Input: part model. Units: mm. Frame: model coordinates. Face numbers are marked on the shaded views. A direction names the side the tool comes from. Give positions to 0.01 mm unless a question says otherwise; leave off trailing zeros. Order: outer loops, then holes, each group sorted by start corner. A loop starts at its lowest first (then second) coordinate and runs counter-clockwise, first axis right, second up.
```python
from build123d import *

# Parameters (mm, degrees)
BOSS_EXTRUDE1_DEPTH = 56.45658
BOSS_EXTRUDE2_DEPTH = 6.2738
BOSS_EXTRUDE3_DEPTH = 6.2738
SKETCH5_R           = 3.1369
CUT_EXTRUDE1_DEPTH  = 22.95576
SKETCH6_R           = 7.05612
CUT_EXTRUDE2_DEPTH  = 53.31968


with BuildPart() as part:
    # Sketch1 → Boss-Extrude1 (new body)
    with BuildSketch(Plane(origin=(0, 0, 0), x_dir=(0, 0, -1), z_dir=(1, 0, 0))):
        with BuildLine():
            Line((10.97788, 10.97788), (10.97788, -10.97788))
            Line((10.97788, -10.97788), (9.4107, -10.97788))
            Line((9.4107, -10.97788), (9.4107, -9.4107))
            Line((9.4107, -9.4107), (0, -9.4107))
            ThreePointArc((0, -9.4107), (-9.4107, 0), (0, 9.4107))
            Line((0, 9.4107), (9.4107, 9.4107))
            Line((9.4107, 9.4107), (9.4107, 10.97788))
            Line((9.4107, 10.97788), (10.97788, 10.97788))
        make_face()
    extrude(amount=-BOSS_EXTRUDE1_DEPTH)

    # Sketch3 → Boss-Extrude2 (add)
    with BuildSketch(Plane(origin=(-1.56718, 0, 0), x_dir=(0, 0, -1), z_dir=(1, 0, 0))):
        with BuildLine():
            Line((9.4107, 10.97788), (0, 10.97788))
            ThreePointArc((0, 10.97788), (-10.97788, 0), (0, -10.97788))
            Line((0, -10.97788), (9.4107, -10.97788))
            Line((9.4107, -10.97788), (9.4107, 10.97788))
        make_face()
    extrude(amount=-BOSS_EXTRUDE2_DEPTH)

    # Sketch4 → Boss-Extrude3 (add)
    with BuildSketch(Plane(origin=(0, 10.97788, 0), x_dir=(1, 0, 0), z_dir=(0, 1, 0))):
        with BuildLine():
            Line((-56.45658, 10.97788), (-65.86728, 10.97788))
            ThreePointArc((-65.86728, 10.97788), (-72.521649786, -5.087189786), (-56.45658, 1.56718))
            Line((-56.45658, 1.56718), (-56.45658, 10.97788))
        make_face()
    boss_extrude3 = extrude(amount=-BOSS_EXTRUDE3_DEPTH)

    # Mirror1: Boss-Extrude3 across plane
    add(boss_extrude3.mirror(Plane.ZX))

    # Sketch5 → Cut-Extrude1 (cut, through all)
    with BuildSketch(Plane(origin=(0, 10.97788, 0), x_dir=(1, 0, 0), z_dir=(0, 1, 0))):
        with Locations((-65.86728, 1.56718)):
            Circle(SKETCH5_R)
    extrude(amount=-CUT_EXTRUDE1_DEPTH, mode=Mode.SUBTRACT)

    # Sketch6 → Cut-Extrude2 (cut)
    with BuildSketch(Plane(origin=(0, 0, 0), x_dir=(0, 0, -1), z_dir=(1, 0, 0))):
        Circle(SKETCH6_R)
    extrude(amount=-CUT_EXTRUDE2_DEPTH, mode=Mode.SUBTRACT)


solid = part.part
```
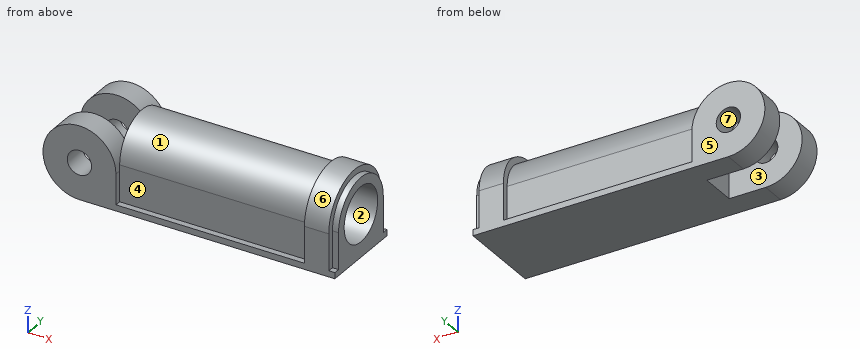
1) Cut plane B-B (y = -1). Return the cut outline in (x, z), then the cut area to 3 significant figures.
2) Reachability of the marked faces 1, 2, 3 and 4 from +Z, -Z, +X, -X, +Y, -Y: full face, straight path, thin tool, end or side. Return the list, or none.
3) Cut plane A-A (x = -15.5). Return the cut outline in (y, z), then the cut area to 3 significant figures.
4) Cut plane D-D (x = -68). Return the cut outline in (y, z), then the cut area to 3 significant figures.
5) Pull-direction query (Z, two-part tool) for the marked faces 5, 6 and 7; classes: pulls with the +Z half, pulls with the -Z half, needs draft (parallel to the pull), parting line crosses it, or undercut.
6) First-contact query: P1, Ø12, axis at x = -52, y = 4.5, coming from the +Z side; P2, Ø4, axis at x = -39.5, y = -7.5, coming from the +Z side; P3, Ø0.8, axis at y = 10, z = -7, coming from the +X side. Flat tips, straight axial feed; report the tip coordinate or a pass-through.
7) Cut plane C-C (z = -5.75). Return the cut outline in (x, y), then the cut area to 3 significant figures.
8) Line query: probe 1 along Y at (x, z) = (-36, 0); probe 2 along Y at (x, z) = (-65, -5); probe 3 along X at (y, z) = (9.5, 1.25). Output: solid intervals per line, ascending.
Geometry says:
1. outline: (-56.46, -10.98) - (0, -10.98) - (0, -6.98) - (-53.32, -6.98) - (-53.32, 6.98) - (0, 6.98) - (0, 9.36) - (-1.57, 9.36) - (-1.57, 10.93) - (-7.84, 10.93) - (-7.84, 9.36) - (-56.46, 9.36) - close
1. area: 413 mm2
2. face 1: +Z
2. face 2: +X
2. face 3: +Z, -Z, -X
2. face 4: +Z, -Y
3. outline: (-10.98, -10.98) - (10.98, -10.98) - (10.98, -9.41) - (9.41, -9.41) - (9.41, 0) arc R9.41 ccw to (-9.41, 0) - (-9.41, -9.41) - (-10.98, -9.41) - close; hole circle Ø14.11 at (0, 0)
3. area: 194 mm2
4. outline: (-10.98, -10.73) - (-4.7, -10.73) - (-4.7, -3.87) - (-10.98, -3.87) - close; (-10.98, 0.73) - (-4.7, 0.73) - (-4.7, 7.6) - (-10.98, 7.6) - close; (4.7, -10.73) - (10.98, -10.73) - (10.98, -3.87) - (4.7, -3.87) - close; (4.7, 0.73) - (10.98, 0.73) - (10.98, 7.6) - (4.7, 7.6) - close
4. area: 172 mm2
5. face 5: needs draft
5. face 6: pulls with the +Z half
5. face 7: undercut
6. P1: stops at z = 9.41
6. P2: stops at z = 7.64
6. P3: stops at x = -1.57
7. outline: (-74.3, -10.98) - (-56.46, -10.98) - (-56.46, -9.41) - (-7.84, -9.41) - (-7.84, -10.98) - (-1.57, -10.98) - (-1.57, -9.41) - (0, -9.41) - (0, -4.09) - (-53.32, -4.09) - (-53.32, 4.09) - (0, 4.09) - (0, 9.41) - (-1.57, 9.41) - (-1.57, 10.98) - (-7.84, 10.98) - (-7.84, 9.41) - (-56.46, 9.41) - (-56.46, 10.98) - (-74.3, 10.98) - (-74.3, 4.7) - (-56.46, 4.7) - (-56.46, -4.7) - (-74.3, -4.7) - close
7. area: 870 mm2
8. probe 1: y = -9.41 to -7.06, 7.06 to 9.41
8. probe 2: y = -10.98 to -4.7, 4.7 to 10.98
8. probe 3: x = -74.85 to -67.25, -64.49 to -56.89, -7.84 to -1.57
